```python
from build123d import *

# Parameters (mm, degrees)
SKETCH1_W           = 22
SKETCH1_H           = 12
SKETCH1_R           = 2.6
BOSS_EXTRUDE1_DEPTH = 3
SKETCH2_W           = 15
SKETCH2_H           = 36
BOSS_EXTRUDE2_DEPTH = 3
FILLET1_R           = 5
FILLET2_R           = 1
SKETCH4_W           = 15
SKETCH4_H           = 34.286255804
BOSS_EXTRUDE3_DEPTH = 12.2
SKETCH9_R           = 1.6
CUT_EXTRUDE1_DEPTH  = 40
SKETCH12_W          = 15
SKETCH12_H          = 40.231404522
BOSS_EXTRUDE5_DEPTH = 3
FILLET3_R           = 5
FILLET4_R           = 5
SKETCH14_W          = 15
SKETCH14_H          = 1.024404938
CUT_EXTRUDE2_DEPTH  = 3
FILLET5_R           = 5


with BuildPart() as part:
    # Sketch1 → Boss-Extrude1 (new body)
    with BuildSketch(Plane(origin=(0, 0, 0), x_dir=(0, 0, -1), z_dir=(1, 0, 0))):
        with Locations((5, 0)):
            Rectangle(SKETCH1_W, SKETCH1_H)
        with Locations((10, 0)):
            Circle(SKETCH1_R, mode=Mode.SUBTRACT)
        Circle(SKETCH1_R, mode=Mode.SUBTRACT)
    extrude(amount=BOSS_EXTRUDE1_DEPTH)

    # Sketch2 → Boss-Extrude2 (add)
    with BuildSketch(Plane(origin=(0, 0, 0), x_dir=(0, 0, -1), z_dir=(1, 0, 0))):
        with Locations((1.5, -24)):
            Rectangle(SKETCH2_W, SKETCH2_H)
    extrude(amount=BOSS_EXTRUDE2_DEPTH)

    # Fillet1
    fillet1_edges = [part.edges().sort_by_distance(p)[0] for p in [
        (1.5, -6, -16),
        (1.5, 6, 6),
        (1.5, 6, -16),
    ]]
    fillet(fillet1_edges, radius=FILLET1_R)

    # Fillet2
    fillet2_edges = [part.edges().sort_by_distance(p)[0] for p in [
        (1.5, -42, 6),
        (1.5, -42, -9),
    ]]
    fillet(fillet2_edges, radius=FILLET2_R)

    # Sketch4 → Boss-Extrude3 (add)
    with BuildSketch(Plane(origin=(3, 0, 0), x_dir=(0, 0, -1), z_dir=(1, 0, 0))):
        with Locations((1.5, -23.856872098)):
            Rectangle(SKETCH4_W, SKETCH4_H)
    extrude(amount=BOSS_EXTRUDE3_DEPTH)

    # Sketch9 → Cut-Extrude1 (cut)
    with BuildSketch(Plane.ZY):
        with Locations((-1.5, -25.546825535)):
            Circle(SKETCH9_R)
        with Locations((-1.5, -15.746825535)):
            Circle(SKETCH9_R)
    extrude(amount=-CUT_EXTRUDE1_DEPTH, mode=Mode.SUBTRACT)

    # Sketch12 → Boss-Extrude5 (add)
    with BuildSketch(Plane.ZY):
        with Locations((-1.5, -55.884297739)):
            Rectangle(SKETCH12_W, SKETCH12_H)
    extrude(amount=BOSS_EXTRUDE5_DEPTH)

    # Fillet3
    # the kernel refuses this fillet: 5 mm, written as the material it adds along each edge
    with BuildSketch(Plane(origin=(0, -35.768595478, -9), x_dir=(0, 1, 0), z_dir=(0, 0, 1))) as fillet3_piece_1:
        with BuildLine():
            CenterArc((4.582575695, 5), FILLET3_R, 203.578178478, 66.421821522)
            Line((0, 3), (-0.091651514, 2.96))
            ThreePointArc((-0.091651514, 2.96), (-0.1, 1.5), (-0.1, 0))
            Line((-0.1, 0), (0, -0.1))
            Line((0, -0.1), (4.582575695, -0.1))
            Line((4.582575695, -0.1), (4.582575695, 0))
        make_face()
    extrude(amount=15)

    # Fillet4
    fillet4_edges = [part.edges().sort_by_distance(p)[0] for p in [
        (-3, -35.768595478, -1.5),
    ]]
    fillet(fillet4_edges, radius=FILLET4_R)

    # Sketch14 → Cut-Extrude2 (cut)
    with BuildSketch(Plane(origin=(3, 0, 0), x_dir=(0, 0, -1), z_dir=(1, 0, 0))):
        with Locations((1.5, -41.512202469)):
            Rectangle(SKETCH14_W, SKETCH14_H)
    extrude(amount=-CUT_EXTRUDE2_DEPTH, mode=Mode.SUBTRACT)

    # Fillet5
    fillet5_edges = [part.edges().sort_by_distance(p)[0] for p in [
        (0, -41, -1.5),
    ]]
    fillet(fillet5_edges, radius=FILLET5_R)


solid = part.part
```
For this review, take the finished solid that the model builds, in its own axes (mm). A direction names the side the tool comes from. Round coordinates to 2 decimals unless told otherwise and drop trailing zeros. Write each loop counter-clockwise with the first axis right and the second up, starting at its lowest first coordinate (ties: lowest second). Pieces come first, ordered by that corner, then holes. Notation, with made-up numbers: (80, -22.5) - (93, -22.5) arc R15 cw to (93, -13.5) - close; hole circle Ø10 at (67, 20.25). An arc over 180 degrees is marked (long way). Put each result on its own line as item: value.
Q1. We need section D-D (x = 4). Give the boundary of the cut face in (y, z), and give its area (3 significant figures).
Solved:
outline: (-41.1, -9) - (-6.71, -9) - (-6.71, 6) - (-41.1, 6) - close; hole circle Ø3.2 at (-25.55, -1.5); hole circle Ø3.2 at (-15.75, -1.5)
area: 500 mm2
Q2. Insertion check: pin 1 Ø1.5 at (x, z) = (5.5, -9) entering from -Y; pin 2 Ø4 at (y, z) = (-2.5, -9.5) entering from +X; pin 3 Ø7.5 at (y, z) = (-58, -5) entering from +X; pin 4 Ø4.5 at (y, z) = (0, -10) entering from -X. Each pin has a flat end and moves straight along its axis. Give the tip position at first contact, or say it passes through.
Solved:
pin 1: stops at y = -41.01
pin 2: stops at x = 3
pin 3: stops at x = 0
pin 4: passes through
Q3. Wall thickness on probe 1 along Y at (x, z) = (7, -1.5); probe 2 along Y at (x, z) = (1.75, -10); probe 3 along Y at (x, z) = (3.25, -0.25): over which ranges is each line inside the solid? List them lowest first.
Solved:
probe 1: y = -41 to -27.15, -23.95 to -17.35, -14.15 to -6.71
probe 2: y = -6 to -2.6, 2.6 to 6
probe 3: y = -41.32 to -26.55, -24.55 to -16.75, -14.75 to -6.71
Q4. We need section B-B (y = 0). Give the boundary of the cut face in (x, z).
Solved:
outline: (0, -16) - (3, -16) - (3, -12.6) - (0, -12.6) - close; (0, -7.4) - (3, -7.4) - (3, -2.6) - (0, -2.6) - close; (0, 2.6) - (3, 2.6) - (3, 6) - (0, 6) - close
Q5. We need section A-A (z = -10). Give the boundary of the cut face in (x, y).
Solved:
outline: (0, -6) - (3, -6) - (3, -2.6) - (0, -2.6) - close; (0, 2.6) - (3, 2.6) - (3, 6) - (0, 6) - close
Q6. We need section C-C (z = -1.5). Give the boundary of the cut face in (x, y).
Solved:
outline: (-3, -76) - (0, -76) - (0, -46) arc R5 cw to (5, -41) - (15.2, -41) - (15.2, -27.15) - (0, -27.15) - (0, -31.19) arc R5 cw to (-1.5, -34.76) arc R5 ccw to (-3, -38.33) - close; (0, -23.95) - (15.2, -23.95) - (15.2, -17.35) - (0, -17.35) - close; (0, -14.15) - (15.2, -14.15) - (15.2, -6.71) - (3, -6.71) - (3, -2.12) - (0, -2.12) - close; (0, 2.12) - (3, 2.12) - (3, 6) - (0, 6) - close
Q7. Mouldability with a two-part tool opening along Y and no side actions: class faces 1 (the face through (1, -43, -2)), 2 (the face through (1.479, 2.578, 0.338)), 3 (the face through (9, -6.714, -1)) as released by +Y, released by -Y, zero draft, split by the parting line, or undercut.
Solved:
face 1: released by -Y
face 2: undercut
face 3: released by +Y
Q8. Machinability: for faces 4 (the face through (3, 0, -5)), 5 (the face through (2, 4, -15)), 6 (the face through (0, -61, -2)), which of the approach directions +Z, -Z, +X, -X, +Y, -Y give a long, thin tool a straight path to every point of the face, cutting with its end or side? Answer none if there is none.
Solved:
face 4: +Z, -Z, +X, +Y
face 5: -Z, +X, -X, +Y
face 6: +Z, -Z, +X, -Y
